```python
from build123d import *

# Parameters (mm, degrees)
F1_DEPTH = 101.6


with BuildPart() as f1:
    # F0 (on Front) → F1 (new body)
    with BuildSketch(Plane.XZ):
        with BuildLine():
            Line((50.8, 101.6), (-76.2, 101.6))
            ThreePointArc((-76.2, 101.6), (-94.160512, 94.160512), (-101.6, 76.2))
            Line((-101.6, 76.2), (-101.6, -50.8))
            ThreePointArc((-101.6, -50.8), (-86.721024, -86.721024), (-50.8, -101.6))
            Line((-50.8, -101.6), (76.2, -101.6))
            ThreePointArc((76.2, -101.6), (94.160512, -94.160512), (101.6, -76.2))
            Line((101.6, -76.2), (101.6, 50.8))
            ThreePointArc((101.6, 50.8), (86.721024, 86.721024), (50.8, 101.6))
        make_face()
    extrude(amount=F1_DEPTH)


solid = f1.part
```
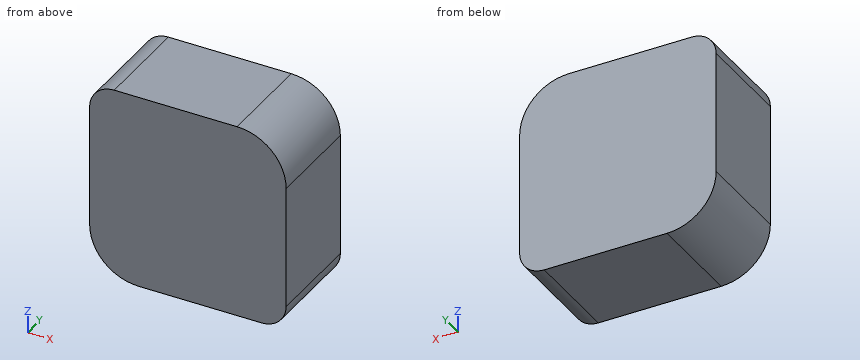
Design review of the part built by this model. Coordinates are the model's own, in mm. Give positions to 0.01 mm unless a question says otherwise; leave off trailing zeros. Loops run counter-clockwise (first coordinate to the right, second up) from the corner with the lowest first, then second, coordinate; pieces in that order, holes last. Notation, with made-up numbers: M -39.75,-32.5 L 15.25,-32.5 A22 ccw 15.25,-11.5 Z; hole C -40,-20.5 d4. An arc over 180 degrees is marked long. Return JSON: item names as keys, results as strings. Group by question number.
Item 1: We need section A-A (y = -14.5). Give the boundary of the cut face in (x, z).
Item 2: For probe 1 along X at (y, z) = (-87, 57); probe 2 along Z at (x, y) = (92, -59); probe 3 along Z at (x, y) = (78.5, -93.5), list the stretches that pass through material, from the lowest coordinate up.
Item 3: We need section C-C (x = -79.5). Give the boundary of the cut face in (y, z), and give its area (3 significant figures).
Item 4: We need section B-B (z = -87). Give the boundary of the cut face in (x, y).
Item 5: Insertion check: pin 1 Ø1 at (x, z) = (-25.5, 50.5) entering from +Y; pin 2 Ø2 at (x, y) = (81, -79) entering from -Z; pin 3 Ø8 at (x, y) = (78.5, -90.5) entering from +Z. Each pin has a flat end and moves straight along its axis. Give the tip position at first contact, or say it passes through.
Output:
{
 "1": {"outline": "M -101.6,-50.8 A50.8 ccw -50.8,-101.6 L 76.2,-101.6 A25.4 ccw 101.6,-76.2 L 101.6,50.8 A50.8 ccw 50.8,101.6 L -76.2,101.6 A25.4 ccw -101.6,76.2 Z"},
 "2": {"probe 1": "x = -101.6 to 101.22", "probe 2": "z = -96.09 to 80.52", "probe 3": "z = -101.5 to 93.38"},
 "3": {"outline": "M -101.6,-92.72 L 0,-92.72 L 0,101.38 L -101.6,101.38 Z", "area": "19,700 mm^2"},
 "4": {"outline": "M -86.44,-101.6 L 99.19,-101.6 L 99.19,0 L -86.44,0 Z"},
 "5": {"pin 1": "stops at y = 0", "pin 2": "stops at z = -101.31", "pin 3": "stops at z = 95.73"}
}
